For this review, take the finished solid that the model builds, in its own axes (mm). Face numbers are marked on the shaded views. A direction names the side the tool comes from. Coordinates: 2 decimals unless noted, no trailing zeros. Order: outer loops, then holes, each group sorted by start corner. A loop starts at its lowest first (then second) coordinate and runs counter-clockwise, first axis right, second up. Notation, with made-up numbers: (51.5, 36) - (110.5, 36) arc R16 ccw to (110.5, 41) - close; hole circle Ø4 at (-28.75, -7). An arc over 180 degrees is marked (long way). One line per item, written item: value. Start each with the question number.
(1) To check wall thickness, follow line 1 along Y through (x, z) = (-16.5, 2.5); line 2 along Y through (x, z) = (12, 0.5); line 3 along X through (y, z) = (5, 1.75). State the ranges of each line that lie inside material, in increasing order.
(2) Clearance check with flat-ended pins moving along their axes: pin 1 (1.8 mm diameter, centred on x = -24.5, y = 2, fed in from -Z); pin 2 (5 mm diameter, centred on x = -17.5, y = -2, fed in from +Z); pin 3 (1 mm diameter, centred on x = 12.5, y = -2.5, fed in from -Z). State where each tip first meets the part, or that it passes through.
(3) Consider section A-A on x = 6.5. Write out the cut boundary in (y, z), then the cut area to 3 significant figures.
(4) Consider section B-B on x = -16. Write out the cut boundary in (y, z), then the cut area to 3 significant figures.
(5) For the marked faces 1 and 2, list the 3-axis set-ups (+Z, -Z, +X, -X, +Y, -Y) from which the entire face can be reached by the end or side of a thin tool; tool diameter is ignored.
```python
from build123d import *

# Parameters (mm, degrees)
BOSS_EXTRUDE1_START = -25.4
BOSS_EXTRUDE1_DEPTH = 3.1242
CUT_EXTRUDE2_DEPTH  = 28.214390217
DRAFT2_ANGLE        = -3
CIRPATTERN3_COUNT   = 4


with BuildPart() as part:
    # Sketch13 → Revolve2 (revolve)
    with BuildSketch(Plane.XY, mode=Mode.PRIVATE) as revolve2_sk:
        Polygon((-25.4, 0), (-25.4, 6.9088), (-25.266671341, 6.9088), (-21.2344, 3.4036), (-8.4582, 3.4036), (-5.419022903, 2.29743), (19.27352, 2.29743), (23.312066741, 1.382457188), (25.4, 0), align=None)
    revolve(revolve2_sk.sketch.rotate(Axis((-25.4, 0, 0), (1, 0, 0)), 180), axis=Axis((-25.4, 0, 0), (1, 0, 0)))


with BuildPart() as body_2:
    # Sketch9 → Boss-Extrude1 (new body)
    with BuildSketch(Plane(origin=(0, 0, 0), x_dir=(0, 0, -1), z_dir=(1, 0, 0)).offset(BOSS_EXTRUDE1_START)):
        Polygon((0.621792, -1.648367869), (0.621792, -3.523488), (-0.621792, -3.523488), (-0.621792, -1.648367869), (-0.933766565, -0.933766565), (-1.648367869, -0.621792), (-3.523488, -0.621792), (-3.523488, 0.621792), (-1.648367869, 0.621792), (-0.933766565, 0.933766565), (-0.621792, 1.648367869), (-0.621792, 3.523488), (0.621792, 3.523488), (0.621792, 1.648367869), (0.933766565, 0.933766565), (1.648367869, 0.621792), (3.523488, 0.621792), (3.523488, -0.621792), (1.648367869, -0.621792), (0.933766565, -0.933766565), align=None)
    extrude(amount=BOSS_EXTRUDE1_DEPTH)

    # Sketch10 → Cut-Extrude2 (cut, symmetric)
    with BuildSketch(Plane.XY):
        Polygon((-24.96566, 3.523488), (-22.2758, 1.907257055), (-22.2758, 3.523488), align=None)
    cut_extrude2 = extrude(amount=CUT_EXTRUDE2_DEPTH, both=True, mode=Mode.SUBTRACT)

    # Draft2
    draft2_faces = [body_2.faces().sort_by_distance(p)[0] for p in [
        (-23.8379, 0.777779282, 1.291067217),
        (-23.8379, 1.291067217, 0.777779282),
        (-23.8379, 1.291067217, -0.777779282),
        (-23.8379, 0.777779282, -1.291067217),
        (-23.8379, -0.777779282, -1.291067217),
        (-23.8379, -1.291067217, -0.777779282),
        (-23.8379, -0.777779282, 1.291067217),
        (-23.8379, -1.291067217, 0.777779282),
    ]]
    draft(draft2_faces, Plane(origin=(-25.4, 0, 0), x_dir=(0, 0, -1), z_dir=(-1, 0, 0)), DRAFT2_ANGLE)

    # CirPattern3: Cut-Extrude2 ×4 about axis
    cirpattern3_axis = Axis((0, 0, 0), (1, 0, 0))
    for i in range(1, CIRPATTERN3_COUNT):
        add(cut_extrude2.rotate(cirpattern3_axis, i * 360 / CIRPATTERN3_COUNT), mode=Mode.SUBTRACT)


with BuildPart() as part_1:
    add(part.part)

    # Combine2: cut body 2
    add(body_2.part, mode=Mode.SUBTRACT)


solid = part_1.part
```
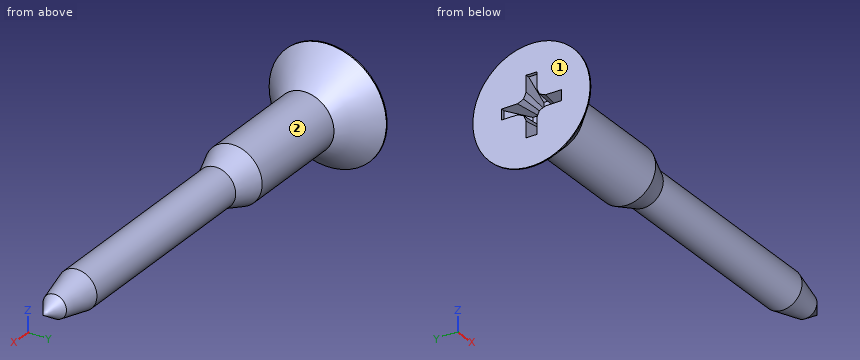
Geometry check:
1. line 1: y = -2.31 to 2.31
1. line 2: y = -2.24 to 2.24
1. line 3: x = -25.4 to -23.41
2. pin 1: stops at z = -6.74
2. pin 2: stops at z = 3.4
2. pin 3: stops at z = -1.13
3. outline: circle Ø4.59 at (0, 0)
3. area: 16.6 mm^2
4. outline: circle Ø6.81 at (0, 0)
4. area: 36.4 mm^2
5. face 1: +Z, -Z, -X, +Y, -Y
5. face 2: +X
